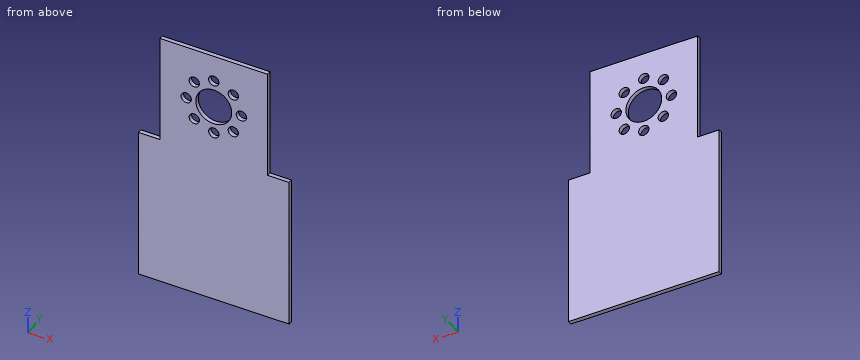
```python
from build123d import *

# Parameters (mm, degrees)
SKETCH1_R           = 1.8288
SKETCH1_R_2         = 6.35
BOSS_EXTRUDE1_DEPTH = 1.5


with BuildPart() as part:
    # Sketch1 → Boss-Extrude1 (new body)
    with BuildSketch(Plane(origin=(0, 0, 0), x_dir=(1, 0, 0), z_dir=(0, 1, 0))):
        Polygon((-21.410875754, -45.056521739), (16.689124246, -45.056521739), (16.689124246, -6.956521739), (24.298964246, -6.956521739), (24.298964246, 46.363158261), (-29.020715754, 46.363158261), (-29.020715754, -6.956521739), (-21.410875754, -6.956521739), align=None)
        with Locations(Location((-9.275672968, -19.091724526, 0), (0, 0, 270))):
            Circle(SKETCH1_R, mode=Mode.SUBTRACT)
        with Locations(Location((-2.360875754, -16.227521739, 0), (0, 0, 270))):
            Circle(SKETCH1_R, mode=Mode.SUBTRACT)
        with Locations(Location((-12.139875754, -26.006521739, 0), (0, 0, 270))):
            Circle(SKETCH1_R, mode=Mode.SUBTRACT)
        with Locations(Location((4.553921459, -19.091724526, 0), (0, 0, 270))):
            Circle(SKETCH1_R, mode=Mode.SUBTRACT)
        with Locations(Location((7.418124246, -26.006521739, 0), (0, 0, 270))):
            Circle(SKETCH1_R, mode=Mode.SUBTRACT)
        with Locations(Location((4.553921459, -32.921318952, 0), (0, 0, 270))):
            Circle(SKETCH1_R, mode=Mode.SUBTRACT)
        with Locations(Location((-2.360875754, -35.785521739, 0), (0, 0, 270))):
            Circle(SKETCH1_R, mode=Mode.SUBTRACT)
        with Locations(Location((-9.275672968, -32.921318952, 0), (0, 0, 270))):
            Circle(SKETCH1_R, mode=Mode.SUBTRACT)
        with Locations(Location((-2.360875754, -26.006521739, 0), (0, 0, 270))):
            Circle(SKETCH1_R_2, mode=Mode.SUBTRACT)
    extrude(amount=BOSS_EXTRUDE1_DEPTH)


solid = part.part
```
The listing builds one solid part. Answer for the finished solid, in the listing's coordinates (mm). Give positions to 0.01 mm unless a question says otherwise; leave off trailing zeros. Order: outer loops, then holes, each group sorted by start corner. A loop starts at its lowest first (then second) coordinate and runs counter-clockwise, first axis right, second up. Notation, with made-up numbers: (21.5, 78.25) -> (67.5, 78.25) arc R21 cw to (67.5, 105.25) -> close; hole circle Ø1 at (-17, 47). An arc over 180 degrees is marked (long way). Answer as CSV lines item,"result". Start each with the question number.
Q1. A cutting plane is placed at B-B (z = 29). Determine the outline of the cut face in (x, y), then the cut area to 3 significant figures.
Q2. A cutting plane is placed at D-D (z = 8.5). Determine the outline of the cut face in (x, y), then the cut area to 4 significant figures.
Q3. A cutting plane is placed at C-C (y = 1.05). Count the separate pieces of the cut face and the enclosed holes in it, then the cut area to 3 significant figures.
Q4. Given pin 1 (6 mm diameter, centred on x = -17.5, z = -33, fed in from -Y); pin 2 (0.8 mm diameter, centred on x = -25.5, y = 1, fed in from +Z), each flat-ended and moving along its own axis, determine where each tip first touches the part or whether it passes through.
Q5. Find the intervals of material crossed by L1, parallel to X at y = 0.2, z = 27.5; L2, parallel to Z at x = -13.5, y = 1.1; L3, parallel to X at y = 0.5, z = 30, in increasing order.
Q6. A cutting plane is placed at A-A (x = -1.5). Determine the outline of the cut face in (y, z).
Results found:
1,outline,"(-21.41, 0) -> (-7.96, 0) -> (-7.96, 1.5) -> (-21.41, 1.5) -> close; (3.24, 0) -> (16.69, 0) -> (16.69, 1.5) -> (3.24, 1.5) -> close"
1,area,"40.3 mm2"
2,outline,"(-21.41, 0) -> (16.69, 0) -> (16.69, 1.5) -> (-21.41, 1.5) -> close"
2,area,"57.15 mm2"
3,separate pieces,"1"
3,enclosed holes,"9"
3,area,"4,080 mm2"
4,pin 1,"y = 0"
4,pin 2,"z = 6.96"
5,L1,"-21.41 to -13.2, -11.08 to -8.53, 3.81 to 6.36, 8.47 to 16.69"
5,L2,"-46.36 to 24.78, 27.23 to 45.06"
5,L3,"-21.41 to -7.3, 2.58 to 16.69"
6,outline,"(0, -46.36) -> (1.5, -46.36) -> (1.5, 14.61) -> (0, 14.61) -> close; (0, 17.84) -> (1.5, 17.84) -> (1.5, 19.72) -> (0, 19.72) -> close; (0, 32.3) -> (1.5, 32.3) -> (1.5, 34.17) -> (0, 34.17) -> close; (0, 37.4) -> (1.5, 37.4) -> (1.5, 45.06) -> (0, 45.06) -> close"
